from build123d import *

# Parameters (mm, degrees)
F0_W     = 177.8
F0_H     = 127
F0_W_2   = 12.7
F0_H_2   = 12.7
F1_DEPTH = 10.16


with BuildPart() as f1:
    # F0 (on Top) → F1 (new body)
    with BuildSketch(Plane.XY):
        Rectangle(F0_W, F0_H)
        with Locations((-69.85, -44.449999)):
            Rectangle(F0_W_2, F0_H_2, mode=Mode.SUBTRACT)
        with Locations((-44.45, -44.45)):
            Rectangle(F0_W_2, F0_H_2, mode=Mode.SUBTRACT)
        with Locations((-19.05, -44.45)):
            Rectangle(F0_W_2, F0_H_2, mode=Mode.SUBTRACT)
        with Locations((-69.85, -19.049999)):
            Rectangle(F0_W_2, F0_H_2, mode=Mode.SUBTRACT)
        with Locations((-44.45, -19.05)):
            Rectangle(F0_W_2, F0_H_2, mode=Mode.SUBTRACT)
        with Locations((-19.05, -19.05)):
            Rectangle(F0_W_2, F0_H_2, mode=Mode.SUBTRACT)
        with Locations((19.05, -44.45)):
            Rectangle(F0_W_2, F0_H_2, mode=Mode.SUBTRACT)
        with Locations((44.45, -44.45)):
            Rectangle(F0_W_2, F0_H_2, mode=Mode.SUBTRACT)
        with Locations((69.865507, -44.449999)):
            Rectangle(F0_W_2, F0_H_2, mode=Mode.SUBTRACT)
        with Locations((19.05, -19.05)):
            Rectangle(F0_W_2, F0_H_2, mode=Mode.SUBTRACT)
        with Locations((44.45, -19.05)):
            Rectangle(F0_W_2, F0_H_2, mode=Mode.SUBTRACT)
        with Locations((69.865507, -19.049999)):
            Rectangle(F0_W_2, F0_H_2, mode=Mode.SUBTRACT)
        with Locations((-69.85, 19.05)):
            Rectangle(F0_W_2, F0_H_2, mode=Mode.SUBTRACT)
        with Locations((-44.45, 19.05)):
            Rectangle(F0_W_2, F0_H_2, mode=Mode.SUBTRACT)
        with Locations((-19.05, 19.05)):
            Rectangle(F0_W_2, F0_H_2, mode=Mode.SUBTRACT)
        with Locations((-69.85, 44.45)):
            Rectangle(F0_W_2, F0_H_2, mode=Mode.SUBTRACT)
        with Locations((-44.45, 44.45)):
            Rectangle(F0_W_2, F0_H_2, mode=Mode.SUBTRACT)
        with Locations((-19.05, 44.45)):
            Rectangle(F0_W_2, F0_H_2, mode=Mode.SUBTRACT)
        with Locations((19.05, 19.05)):
            Rectangle(F0_W_2, F0_H_2, mode=Mode.SUBTRACT)
        with Locations((44.45, 19.05)):
            Rectangle(F0_W_2, F0_H_2, mode=Mode.SUBTRACT)
        with Locations((69.865507, 19.050001)):
            Rectangle(F0_W_2, F0_H_2, mode=Mode.SUBTRACT)
        with Locations((19.05, 44.45)):
            Rectangle(F0_W_2, F0_H_2, mode=Mode.SUBTRACT)
        with Locations((44.45, 44.45)):
            Rectangle(F0_W_2, F0_H_2, mode=Mode.SUBTRACT)
        with Locations((69.865507, 44.450001)):
            Rectangle(F0_W_2, F0_H_2, mode=Mode.SUBTRACT)
    extrude(amount=F1_DEPTH)


solid = f1.part
Design review of the part built by this model. Coordinates are the model's own, in mm. A direction names the side the tool comes from. Round coordinates to 2 decimals unless told otherwise and drop trailing zeros. Write each loop counter-clockwise with the first axis right and the second up, starting at its lowest first coordinate (ties: lowest second). Pieces come first, ordered by that corner, then holes.
Item 1: For faces 1 (the flat face through (-1, 1, 10.16)), 2 (the flat face through (25.4, 44, 5)), list the 3-axis set-ups (+Z, -Z, +X, -X, +Y, -Y) from which the entire face can be reached by the end or side of a thin tool; tool diameter is ignored.
Item 2: Consider section B-B on x = 71. Give the boundary of the cut face in (y, z), and give its area (3 significant figures).
Item 3: For pin 1 Ø3 at (x, y) = (66.5, -42) entering from +Z, flat-tipped, find the tip position at first contact; note if it passes through.
Item 4: Consider section A-A on y = -43.5. Give the boundary of the cut face in (x, z), and give its area (3 significant figures).
Item 5: Draft analysis for pull direction X (two halves, no side actions). For faces 3 (the flat face through (12.7, 19, 5)), 4 (the flat face through (-1, 1, 0)), state which applies: released by +X, released by -X, zero draft, split by the parting line, or undercut.
Item 6: Consider section C-C on z = 5.25. Count the separate pieces of the cut face and the enclosed holes in it, and give its area (3 significant figures).
Item 7: Wall thickness on L1, parallel to Y at x = 18, z = 9.75: over which ranges is the line inside the solid? List them lowest first.
Check values:
1. face 1: +Z, +X, -X, +Y, -Y
1. face 2: +Z, -Z
2. outline: (-63.5, 0) - (-50.8, 0) - (-50.8, 10.16) - (-63.5, 10.16) - close; (-38.1, 0) - (-25.4, 0) - (-25.4, 10.16) - (-38.1, 10.16) - close; (-12.7, 0) - (12.7, 0) - (12.7, 10.16) - (-12.7, 10.16) - close; (25.4, 0) - (38.1, 0) - (38.1, 10.16) - (25.4, 10.16) - close; (50.8, 0) - (63.5, 0) - (63.5, 10.16) - (50.8, 10.16) - close
2. area: 774 mm2
3. pin 1: passes through
4. outline: (-88.9, 0) - (-76.2, 0) - (-76.2, 10.16) - (-88.9, 10.16) - close; (-63.5, 0) - (-50.8, 0) - (-50.8, 10.16) - (-63.5, 10.16) - close; (-38.1, 0) - (-25.4, 0) - (-25.4, 10.16) - (-38.1, 10.16) - close; (-12.7, 0) - (12.7, 0) - (12.7, 10.16) - (-12.7, 10.16) - close; (25.4, 0) - (38.1, 0) - (38.1, 10.16) - (25.4, 10.16) - close; (50.8, 0) - (63.52, 0) - (63.52, 10.16) - (50.8, 10.16) - close; (76.22, 0) - (88.9, 0) - (88.9, 10.16) - (76.22, 10.16) - close
4. area: 1,030 mm2
5. face 3: undercut
5. face 4: zero draft
6. separate pieces: 1
6. enclosed holes: 24
6. area: 18,700 mm2
7. L1: y = -63.5 to -50.8, -38.1 to -25.4, -12.7 to 12.7, 25.4 to 38.1, 50.8 to 63.5
